Source: three-view drawing plus pictorial views. Frame: mm from the lowest corner of the part. A direction names the side the tool comes from. Give positions to 0.01 mm unless a question says otherwise; leave off trailing zeros. Loops run counter-clockwise (first coordinate to the right, second up) from the corner with the lowest first, then second, coordinate; pieces in that order, holes last. Notation, with made-up numbers: (13, -15) - (53, -15) arc R19 ccw to (53, 4) - close; hole circle Ø9 at (75, -35.5). An arc over 180 degrees is marked (long way). Write each question's results on one line, items separated by ' | '. Start each with the question number.
(1) Cut plane B-B on x = 20. Return the cut outline in (y, z), then the cut area to 3 significant figures.
(2) Contact query for flat-ended pins moving along their axis: pin 1 (3 mm diameter, centred on x = 16.5, z = 35, fed in from -Y); pin 2 (9 mm diameter, centred on x = 20, z = 30, fed in from -Y). Output: stop coordinate, or through.
(3) Cut plane A-A on z = 10. Return the cut outline in (x, y), then the cut area to 3 significant figures.
(4) Reachability of the marked faces 4 and 5 from +Z, -Z, +X, -X, +Y, -Y: full face, straight path, thin tool, end or side. Return the list, or none.
(5) Material intervals for line 1 along Z through (x, y) = (20, 14.75); line 2 along Y through (x, z) = (27.75, 12); line 3 along Z through (x, y) = (7.75, 12), sorted ascending. Write a range as [from, to].
(6) Cut plane D-D on z = 30. Return the cut outline in (x, y), then the cut area to 3 significant figures.
(7) Pull-direction query (Z, two-part tool) for the marked faces 1, 2 and 3; classes: pulls with the +Z half, pulls with the -Z half, needs draft (parallel to the pull), parting line crosses it, or undercut.
(8) Cut plane C-C on y = 7.5. Return the cut outline in (x, z), then the cut area to 3 significant figures.
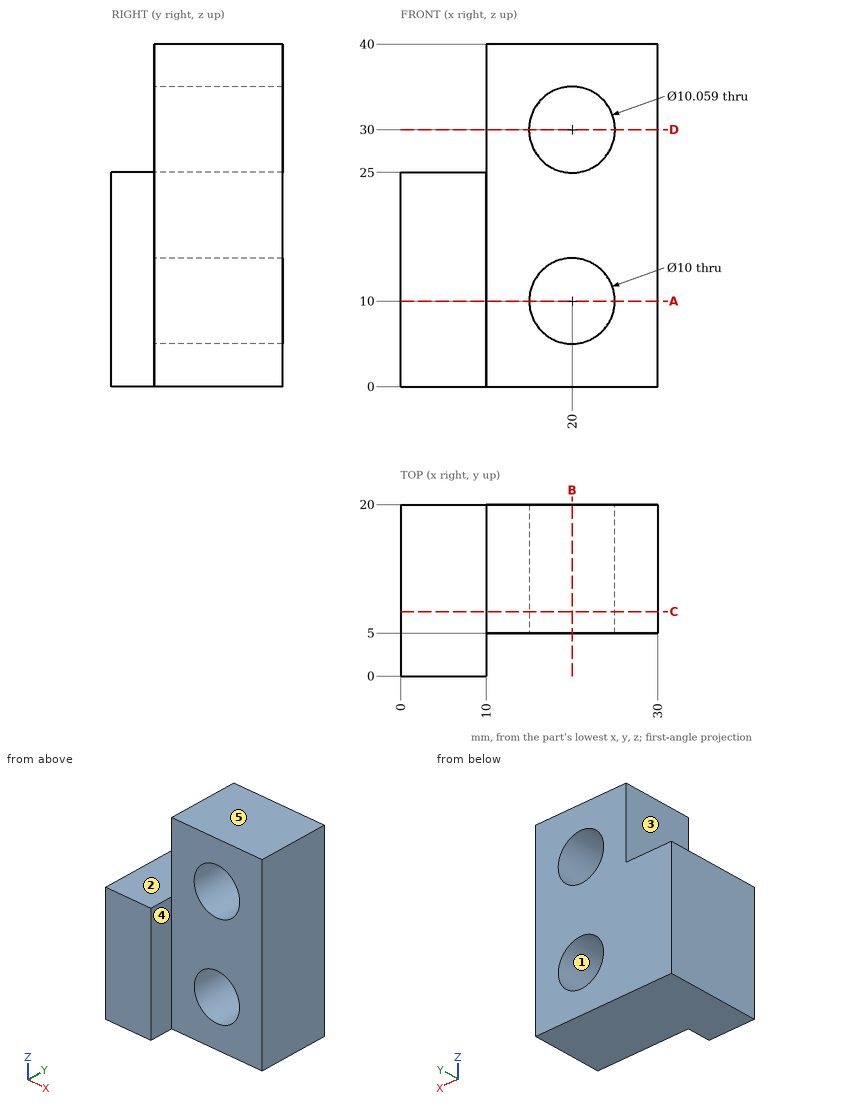
Ans:
1) outline: (5, 0) - (20, 0) - (20, 5) - (5, 5) - close; (5, 15) - (20, 15) - (20, 24.97) - (5, 24.97) - close; (5, 35.03) - (20, 35.03) - (20, 40) - (5, 40) - close | area: 299 mm^2
2) pin 1: y = 5 | pin 2: through
3) outline: (0, 0) - (10, 0) - (10, 5) - (15, 5) - (15, 20) - (0, 20) - close; (25, 5) - (30, 5) - (30, 20) - (25, 20) - close | area: 350 mm^2
4) face 4: +Z, -Z, +X, -Y | face 5: +Z, +X, -X, +Y, -Y
5) line 1: [0, 5], [15, 24.97], [35.03, 40] | line 2: [5, 20] | line 3: [0, 25]
6) outline: (10, 5) - (14.97, 5) - (14.97, 20) - (10, 20) - close; (25.03, 5) - (30, 5) - (30, 20) - (25.03, 20) - close | area: 149 mm^2
7) face 1: undercut | face 2: pulls with the +Z half | face 3: needs draft
8) outline: (0, 0) - (30, 0) - (30, 40) - (10, 40) - (10, 25) - (0, 25) - close; hole circle Ø10.06 at (20, 30); hole circle Ø10 at (20, 10) | area: 892 mm^2
